from build123d import *

# Parameters (mm, degrees)
SKETCH1_R               = 5
BOSS_EXTRUDE1_DEPTH     = 9
SKETCH2_R               = 6
BOSS_EXTRUDE2_DEPTH     = 4.5
SKETCH3_R               = 3
CUT_EXTRUDE1_DEPTH      = 1
CUT_EXTRUDE1_DEPTH_BACK = 14.5


with BuildPart() as part:
    # Sketch1 → Boss-Extrude1 (new body)
    with BuildSketch(Plane(origin=(0, 0, 0), x_dir=(1, 0, 0), z_dir=(0, 1, 0))):
        Circle(SKETCH1_R)
    extrude(amount=BOSS_EXTRUDE1_DEPTH)

    # Sketch2 → Boss-Extrude2 (add)
    with BuildSketch(Plane(origin=(0, 9, 0), x_dir=(1, 0, 0), z_dir=(0, 1, 0))):
        Circle(SKETCH2_R)
    extrude(amount=BOSS_EXTRUDE2_DEPTH)

    # Sketch3 → Cut-Extrude1 (cut, two sides)
    with BuildSketch(Plane(origin=(0, 13.5, 0), x_dir=(1, 0, 0), z_dir=(0, 1, 0))) as cut_extrude1_sk:
        Circle(SKETCH3_R)
    extrude(amount=CUT_EXTRUDE1_DEPTH, mode=Mode.SUBTRACT)
    extrude(cut_extrude1_sk.sketch, amount=-CUT_EXTRUDE1_DEPTH_BACK, mode=Mode.SUBTRACT)


solid = part.part
The model under review builds one solid part; all positions refer to its coordinate system, in mm. A direction names the side the tool comes from. Round coordinates to 2 decimals unless told otherwise and drop trailing zeros. Write each loop counter-clockwise with the first axis right and the second up, starting at its lowest first coordinate (ties: lowest second). Pieces come first, ordered by that corner, then holes. Notation, with made-up numbers: (39.5, 76) -> (55.5, 76) arc R28 cw to (55.5, 108) -> close; hole circle Ø1 at (2.25, -5). An arc over 180 degrees is marked (long way). Answer as a JSON object with one key per item and string values.
1. Machinability: for faces 1 (the face through (-4, 9, -4)), 2 (the face through (-6, 11, 0)), which of the approach directions +Z, -Z, +X, -X, +Y, -Y give a long, thin tool a straight path to every point of the face, cutting with its end or side? Answer none if there is none.
Results found:
{"face 1": "-Y", "face 2": "+Y, -Y"}
2. We need section A-A on x = 0. State the section outline as (y, z) points, and give its area (3 significant figures).
Results found:
{"outline": "(0, -5) -> (9, -5) -> (9, -6) -> (13.5, -6) -> (13.5, -3) -> (0, -3) -> close; (0, 3) -> (13.5, 3) -> (13.5, 6) -> (9, 6) -> (9, 5) -> (0, 5) -> close", "area": "63.0 mm^2"}
3. We need section B-B on z = 1.75. State the section outline as (x, y) points.
Results found:
{"outline": "(-5.74, 9) -> (-4.68, 9) -> (-4.68, 0) -> (-2.44, 0) -> (-2.44, 13.5) -> (-5.74, 13.5) -> close; (2.44, 0) -> (4.68, 0) -> (4.68, 9) -> (5.74, 9) -> (5.74, 13.5) -> (2.44, 13.5) -> close"}
4. We need section D-D on x = -3.5. State the section outline as (y, z) points.
Results found:
{"outline": "(0, -3.57) -> (9, -3.57) -> (9, -4.87) -> (13.5, -4.87) -> (13.5, 4.87) -> (9, 4.87) -> (9, 3.57) -> (0, 3.57) -> close"}
5. Clearance check with flat-ended pins moving along their axes: pin 1 (1.5 mm diameter, centred on x = -3.5, y = 6.5, fed in from -Z); pin 2 (4 mm diameter, centred on y = 11, z = 3.5, fed in from +X); pin 3 (6 mm diameter, centred on y = 4.5, z = 2.5, fed in from +X). State where each tip first meets the part, or that it passes through.
Results found:
{"pin 1": "stops at z = -4.18", "pin 2": "stops at x = 5.81", "pin 3": "stops at x = 5"}
6. We need section C-C on y = 3.5. State the section outline as (x, z) points.
Results found:
{"outline": "circle Ø10 at (0, 0); hole circle Ø6 at (0, 0)"}
7. The part is to be moulded in two halves that separate along Z. For faces 3 (the face through (-3, 7, 0)), 4 (the face through (-3, 13.5, 1)), 5 (the face through (-1.08, 4.44, 4.88)), say which applies: pulls with the +Z half, pulls with the -Z half, needs draft (parallel to the pull), parting line crosses it, or undercut.
Results found:
{"face 3": "undercut", "face 4": "needs draft", "face 5": "parting line crosses it"}
8. To check wall thickness, follow line 1 along X through (y, z) = (10.5, 0); line 2 along X through (y, z) = (4.25, 0). State the ranges of each line that lie inside material, in increasing order.
Results found:
{"line 1": "x = -6 to -3, 3 to 6", "line 2": "x = -5 to -3, 3 to 5"}
